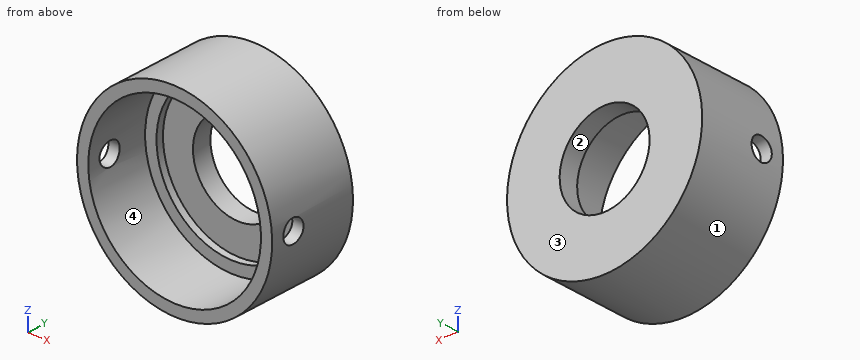
from build123d import *

# Parameters (mm, degrees)
SKETCH1_R               = 20.66925
BOSS_EXTRUDE1_DEPTH     = 19.05
SKETCH2_R               = 18.288
CUT_EXTRUDE1_DEPTH      = 13.3985
SKETCH3_R               = 9.525
CUT_EXTRUDE2_DEPTH      = 35.890375337
SKETCH4_R               = 15.875
CUT_EXTRUDE3_DEPTH      = 1.524
CUT_EXTRUDE4_DEPTH      = 35.890375337
CUT_EXTRUDE4_DEPTH_BACK = 35.890375337
SKETCH5_R               = 2.38125


with BuildPart() as part:
    # Sketch1 → Boss-Extrude1 (new body)
    with BuildSketch(Plane(origin=(0, 0, 0), x_dir=(1, 0, 0), z_dir=(0, 1, 0))):
        with Locations(Location((0, 0, 0), (0, 0, 270))):
            Circle(SKETCH1_R)
    extrude(amount=-BOSS_EXTRUDE1_DEPTH)

    # Sketch2 → Cut-Extrude1 (cut)
    with BuildSketch(Plane.XZ.offset(19.05)):
        with Locations(Location((0, 0, 0), (0, 0, 270))):
            Circle(SKETCH2_R)
    extrude(amount=-CUT_EXTRUDE1_DEPTH, mode=Mode.SUBTRACT)

    # Sketch3 → Cut-Extrude2 (cut, through all)
    with BuildSketch(Plane(origin=(0, 0, 0), x_dir=(1, 0, 0), z_dir=(0, 1, 0))):
        with Locations(Location((0, 0, 0), (0, 0, 270))):
            Circle(SKETCH3_R)
    extrude(amount=-CUT_EXTRUDE2_DEPTH, mode=Mode.SUBTRACT)

    # Sketch4 → Cut-Extrude3 (cut)
    with BuildSketch(Plane.XZ.offset(5.6515)):
        with Locations(Location((0, 0, 0), (0, 0, 270))):
            Circle(SKETCH4_R)
    extrude(amount=-CUT_EXTRUDE3_DEPTH, mode=Mode.SUBTRACT)

    # Sketch5 → Cut-Extrude4 (cut, two sides: drawn at the far end of the back side and taken through both)
    with BuildSketch(Plane(origin=(0, 0, 0), x_dir=(0, 0, -1), z_dir=(1, 0, 0)).offset(-CUT_EXTRUDE4_DEPTH_BACK)):
        with Locations((0, -14.0335)):
            Circle(SKETCH5_R)
    extrude(amount=CUT_EXTRUDE4_DEPTH + CUT_EXTRUDE4_DEPTH_BACK, mode=Mode.SUBTRACT)


solid = part.part
Read the model definition and answer for the solid it produces. Units are mm, in the model's axes. Face numbers are marked on the shaded views. Give positions to 0.01 mm unless a question says otherwise; leave off trailing zeros. Write each loop counter-clockwise with the first axis right and the second up, starting at its lowest first coordinate (ties: lowest second). Pieces come first, ordered by that corner, then holes. Notation, with made-up numbers: (88, 47.5) - (94, 47.5) arc R22 cw to (94, 65.5) - close; hole circle Ø2 at (51.5, 65.25). An arc over 180 degrees is marked (long way). Use CSV: the item, a comma, the result in double quotes. Start each with the question number.
(1) Find section C-C (y = -15.75). Give the vertices of the cut face in (x, z), plus the area to 3 significant figures.
(2) Determine the mould class of the marked faces 1, 2, 3 and 4 for opening direction X: +X half, -X half, draft (parallel to the pull), parting line (faces both ways), or undercut.
(3) Find section D-D (z = -5.5). Give the vertices of the cut face in (x, y).
(4) Given P1, Ø22, axis at x = 0, z = 0, coming from the -Y side; P2, Ø1, axis at x = 4, y = -10, coming from the -Z side; P3, Ø8, axis at x = -11.5, z = 7, coming from the -Y side, each flat-ended and moving along its own axis, determine where each tip first touches the part or whether it passes through.
(5) Find section A-A (z = 0). Count the separate pieces of the cut face and the enclosed holes in it, plus the area to 3 significant figures.
(6) Consider line 1 along X through (y, z) = (-5.3, 0) (3 decimals); line 2 along X through (y, z) = (-17, -0.5); line 3 along Y through (x, z) = (19.1, 0). Determine where each line is inside the solid, lowest interval first.
Findings below:
1,outline,"(-20.6, -1.65) arc R20.67 ccw to (20.6, -1.65) - (18.21, -1.65) arc R18.29 cw to (-18.21, -1.65) - close; (-20.6, 1.65) - (-18.21, 1.65) arc R18.29 cw to (18.21, 1.65) - (20.6, 1.65) arc R20.67 ccw to start"
1,area,"276 mm2"
2,face 1,"parting line"
2,face 2,"undercut"
2,face 3,"draft"
2,face 4,"undercut"
3,outline,"(-19.92, -19.05) - (-17.44, -19.05) - (-17.44, -5.65) - (-14.89, -5.65) - (-14.89, -4.13) - (-7.78, -4.13) - (-7.78, 0) - (-19.92, 0) - close; (7.78, -4.13) - (14.89, -4.13) - (14.89, -5.65) - (17.44, -5.65) - (17.44, -19.05) - (19.92, -19.05) - (19.92, 0) - (7.78, 0) - close"
4,P1,"y = -4.13"
4,P2,"z = -20.37"
4,P3,"y = -5.65"
5,separate pieces,"4"
5,enclosed holes,"0"
5,area,"148 mm2"
6,line 1,"-20.669 to -15.875, 15.875 to 20.669"
6,line 2,"-20.66 to -18.28, 18.28 to 20.66"
6,line 3,"-19.05 to -16.41, -11.65 to 0"
